Model file for the job. Use its own axes, mm. A direction names the side the tool comes from. Round coordinates to 2 decimals unless told otherwise and drop trailing zeros. Write each loop counter-clockwise with the first axis right and the second up, starting at its lowest first coordinate (ties: lowest second). Pieces come first, ordered by that corner, then holes.
```python
from build123d import *

# Parameters (mm, degrees)
SKETCH1_W                               = 150
SKETCH1_H                               = 100
BOSS_EXTRUDE1_DEPTH                     = 20
CBORE_FOR_M5_HEX_HEAD_BOLT1_D           = 5.5
CBORE_FOR_M5_HEX_HEAD_BOLT1_DEPTH       = 15
CBORE_FOR_M5_HEX_HEAD_BOLT1_CBORE_D     = 12.24
CBORE_FOR_M5_HEX_HEAD_BOLT1_CBORE_DEPTH = 3.58
CBORE_FOR_M5_HEX_HEAD_BOLT1_TIP         = 1.652366702
SHELL1_START                            = 1.4
SHELL1_OUTLINE_W                        = 147.2
SHELL1_OUTLINE_H                        = 97.2
SHELL1_OUTLINE_R                        = 7.52
SHELL1_DEPTH                            = 17.2
SHELL1_2_OUTLINE_R                      = 7.52
SHELL1_2_OUTLINE_R_2                    = 4.15
SHELL1_2_DEPTH                          = 13.62
SHELL1_3_OUTLINE_R                      = 4.15
SHELL1_3_DEPTH                          = 0.314346442


with BuildPart() as part:
    # Sketch1 → Boss-Extrude1 (new body)
    with BuildSketch(Plane(origin=(0, 0, 0), x_dir=(1, 0, 0), z_dir=(0, 1, 0))):
        Rectangle(SKETCH1_W, SKETCH1_H)
    extrude(amount=BOSS_EXTRUDE1_DEPTH)

    # CBORE for M5 Hex Head Bolt1
    with Locations(Plane(origin=(0, 20, 0), x_dir=(1, 0, 0), z_dir=(0, 1, 0))):
        with Locations((60, 0), (60, 32), (60, -32)):
            CounterBoreHole(CBORE_FOR_M5_HEX_HEAD_BOLT1_D / 2, CBORE_FOR_M5_HEX_HEAD_BOLT1_CBORE_D / 2, CBORE_FOR_M5_HEX_HEAD_BOLT1_CBORE_DEPTH, depth=CBORE_FOR_M5_HEX_HEAD_BOLT1_DEPTH)
            with Locations((0, 0, -(CBORE_FOR_M5_HEX_HEAD_BOLT1_DEPTH + CBORE_FOR_M5_HEX_HEAD_BOLT1_TIP / 2))):  # 118° drill point
                Cone(0, CBORE_FOR_M5_HEX_HEAD_BOLT1_D / 2, CBORE_FOR_M5_HEX_HEAD_BOLT1_TIP, mode=Mode.SUBTRACT)

    # Shell1: read off the stored shape, not the designer's step
    # Shell1 outline → Shell1 (cut)
    with BuildSketch(Plane(origin=(0, 0, 0), x_dir=(1, 0, 0), z_dir=(0, 1, 0)).offset(SHELL1_START)):
        Rectangle(SHELL1_OUTLINE_W, SHELL1_OUTLINE_H)
        with Locations((60, -32)):
            Circle(SHELL1_OUTLINE_R, mode=Mode.SUBTRACT)
        with Locations((60, 0)):
            Circle(SHELL1_OUTLINE_R, mode=Mode.SUBTRACT)
        with Locations((60, 32)):
            Circle(SHELL1_OUTLINE_R, mode=Mode.SUBTRACT)
    extrude(amount=SHELL1_DEPTH, mode=Mode.SUBTRACT)

    # Shell1 2 outline → Shell1 2 (cut)
    # profile 1 of 3: a face of its own
    with BuildSketch(Plane(origin=(0, 0, 0), x_dir=(1, 0, 0), z_dir=(0, 1, 0)).offset(SHELL1_START)):
        with Locations((60, -32)):
            Circle(SHELL1_2_OUTLINE_R)
        with Locations((60, -32)):
            Circle(SHELL1_2_OUTLINE_R_2, mode=Mode.SUBTRACT)
    # profile 2 of 3: a face of its own
    with BuildSketch(Plane(origin=(0, 0, 0), x_dir=(1, 0, 0), z_dir=(0, 1, 0)).offset(SHELL1_START)):
        with Locations((60, 32)):
            Circle(SHELL1_2_OUTLINE_R)
        with Locations((60, 32)):
            Circle(SHELL1_2_OUTLINE_R_2, mode=Mode.SUBTRACT)
    # profile 3 of 3: a face of its own
    with BuildSketch(Plane(origin=(0, 0, 0), x_dir=(1, 0, 0), z_dir=(0, 1, 0)).offset(SHELL1_START)):
        with Locations((60, 0)):
            Circle(SHELL1_2_OUTLINE_R)
        with Locations((60, 0)):
            Circle(SHELL1_2_OUTLINE_R_2, mode=Mode.SUBTRACT)
    extrude(amount=SHELL1_2_DEPTH, mode=Mode.SUBTRACT)

    # Shell1 3 outline → Shell1 3 (cut)
    with BuildSketch(Plane(origin=(0, 0, 0), x_dir=(1, 0, 0), z_dir=(0, 1, 0)).offset(SHELL1_START)):
        with Locations((60, -32)):
            Circle(SHELL1_3_OUTLINE_R)
        with Locations((60, 32)):
            Circle(SHELL1_3_OUTLINE_R)
        with Locations((60, 0)):
            Circle(SHELL1_3_OUTLINE_R)
    extrude(amount=SHELL1_3_DEPTH, mode=Mode.SUBTRACT)

    # Shell1 4 outline → Shell1 4 (revolve, cut)
    with BuildSketch(Plane(origin=(60, 0, 32), x_dir=(1, 0, 0), z_dir=(0, 0, 1))):
        Polygon((4.15, 4.207918111), (0, 1.714346542), (4.15, 1.714346442), align=None)
    revolve(axis=Axis((60, 0, 32), (0, 1, 0)), mode=Mode.SUBTRACT)

    # Shell1 5 outline → Shell1 5 (revolve, cut)
    with BuildSketch(Plane(origin=(60, 0, -32), x_dir=(1, 0, 0), z_dir=(0, 0, 1))):
        Polygon((4.15, 4.207918111), (0, 1.714346542), (4.15, 1.714346442), align=None)
    revolve(axis=Axis((60, 0, -32), (0, 1, 0)), mode=Mode.SUBTRACT)

    # Shell1 6 outline → Shell1 6 (revolve, cut)
    with BuildSketch(Plane(origin=(60, 0, 0), x_dir=(1, 0, 0), z_dir=(0, 0, 1))):
        Polygon((4.15, 4.207918111), (0, 1.714346542), (4.15, 1.714346442), align=None)
    revolve(axis=Axis((60, 0, 0), (0, 1, 0)), mode=Mode.SUBTRACT)


solid = part.part
```
1) Pull direction X, two halves, no side cores. Call faces 1 (the face through (75, 10, 1)), 2 (the face through (-75, 10, 1)), 3 (the face through (59.523, 3.635, -0.021)): released by +X, released by -X, zero draft, split by the parting line, or undercut.
2) Cut at B-B on x = 47.5. List the corners of the cut face in (y, z).
3) Wall check: probe 1 along X at (y, z) = (10.5, 32); probe 2 along X at (y, z) = (17.65, -32); probe 3 along Z at (x, y) = (-5.5, 8.75). Give the ranges that are in metal, low to high.
4) Cut at A-A on y = 7.75. List the corners of the cut face in (x, z).
5) Flat gauge pins, fed straight in: pin 1 Ø10 at (x, z) = (61, 33.5) entering from +Y; pin 2 Ø3.5 at (x, z) = (62.5, -31.5) entering from +Y. Where does each tip first touch, or does it go through?
6) Cut at C-C on z = -9.5. List the corners of the cut face in (x, y), and give its area (3 significant figures).
7) Which spindle directions (+Z, -Z, +X, -X, +Y, -Y) get a long thin tool onto all of the face, cutting with end or side? Do faces 4 (the face through (55.14, 18.24, 35.72)), 5 (the face through (60.61, 2.11, 0.25)). Say none if no direction does.
Result sheet:
1. face 1: released by +X
1. face 2: released by -X
1. face 3: undercut
2. outline: (0, -50) - (20, -50) - (20, 50) - (0, 50) - close; hole (1.4, -48.6) - (18.6, -48.6) - (18.6, 48.6) - (1.4, 48.6) - close
3. probe 1: x = -75 to -73.6, 55.85 to 57.25, 62.75 to 64.15, 73.6 to 75
3. probe 2: x = -75 to -73.6, 52.48 to 53.88, 66.12 to 67.52, 73.6 to 75
3. probe 3: z = -50 to -48.6, 48.6 to 50
4. outline: (-75, -50) - (75, -50) - (75, 50) - (-75, 50) - close; circle Ø8.3 at (60, -32); circle Ø8.3 at (60, 0); circle Ø8.3 at (60, 32); hole (-73.6, -48.6) - (73.6, -48.6) - (73.6, 48.6) - (-73.6, 48.6) - close; hole circle Ø5.5 at (60, -32); hole circle Ø5.5 at (60, 0); hole circle Ø5.5 at (60, 32)
5. pin 1: stops at y = 20
5. pin 2: stops at y = 16.42
6. outline: (-75, 0) - (75, 0) - (75, 20) - (-75, 20) - close; hole (-73.6, 1.4) - (73.6, 1.4) - (73.6, 18.6) - (-73.6, 18.6) - close
6. area: 468 mm2
7. face 4: +Y
7. face 5: none
